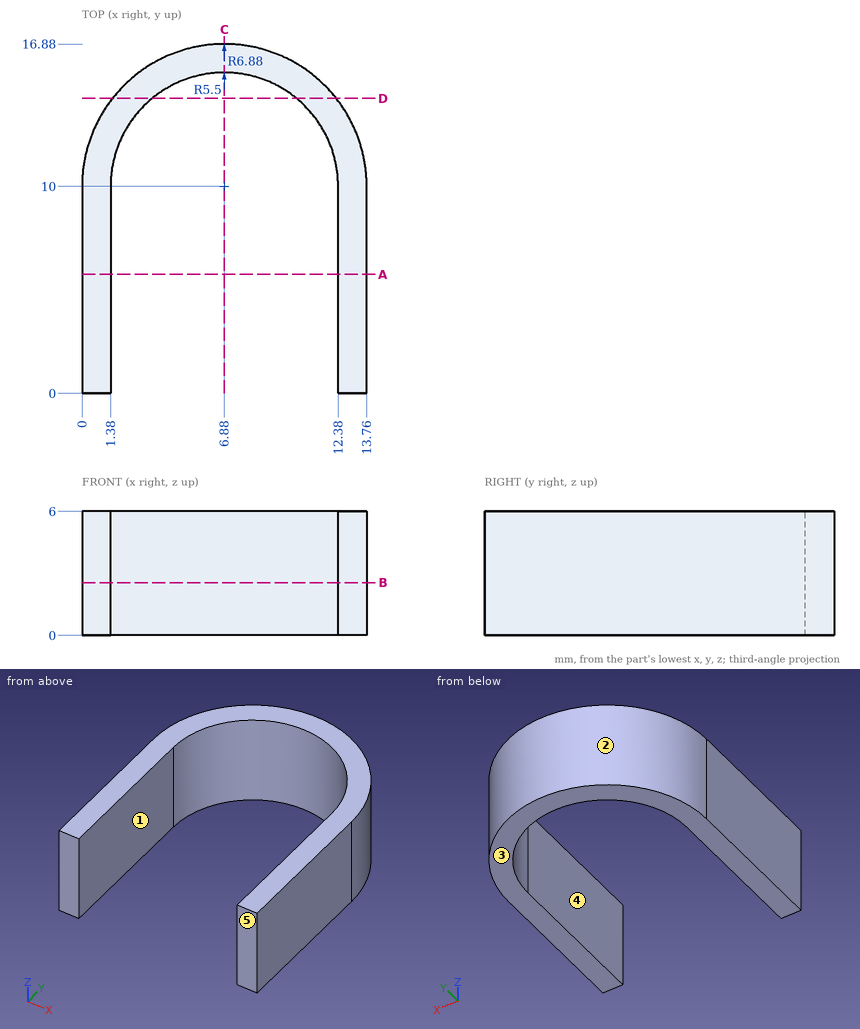
Input: dimensioned drawing with shaded views. Units: mm. Origin: part minimum x, y, z. A direction names the side the tool comes from. Coordinates: 2 decimals unless noted, no trailing zeros. Order: outer loops, then holes, each group sorted by start corner. A loop starts at its lowest first (then second) coordinate and runs counter-clockwise, first axis right, second up. Notation, with made-up numbers: (56, 60.5) -> (108, 60.5) arc R21 cw to (108, 89.5) -> close; hole circle Ø5 at (-6, -26). An arc over 180 degrees is marked (long way). Answer in a Markdown table with one row per item.
Item 1: Section C-C on x = 6.88. Output: boundary loops of the cut face in (y, z).
Return value:
| item | result |
|---|---|
| outline | (15.5, 0) -> (16.88, 0) -> (16.88, 6) -> (15.5, 6) -> close |
Item 2: Contact query for a flat-ended pin moving along its axis: P1, Ø2, axis at x = 10, z = 1, coming from the +Y side. Output: stop coordinate, or through.
Return value:
| item | result |
|---|---|
| P1 | stops at y = 16.55 |
Item 3: Section B-B on z = 2.55. Output: boundary loops of the cut face in (x, y), plus the area to 3 significant figures.
Return value:
| item | result |
|---|---|
| outline | (0, 0) -> (1.38, 0) -> (1.38, 10) arc R5.5 cw to (12.38, 10) -> (12.38, 0) -> (13.76, 0) -> (13.76, 10) arc R6.88 ccw to (0, 10) -> close |
| area | 54.4 mm² |
Item 4: Section D-D on y = 14.25. Output: boundary loops of the cut face in (x, z).
Return value:
| item | result |
|---|---|
| outline | (1.47, 0) -> (3.39, 0) -> (3.39, 6) -> (1.47, 6) -> close; (10.37, 0) -> (12.29, 0) -> (12.29, 6) -> (10.37, 6) -> close |
Item 5: Access query for the marked faces 4 and 5. Directions: +Z, -Z, +X, -X, +Y, -Y. A direction counts if a zero-diameter tool reaches every point of the face in a straight line with its end or side. Return the directions, or none.
Return value:
| item | result |
|---|---|
| face 4 | +Z, -Z, -Y |
| face 5 | +Z, -Z, +X, -X, -Y |
Item 6: Section A-A on y = 5.75. Output: boundary loops of the cut face in (x, z).
Return value:
| item | result |
|---|---|
| outline | (0, 0) -> (1.38, 0) -> (1.38, 6) -> (0, 6) -> close; (12.38, 0) -> (13.76, 0) -> (13.76, 6) -> (12.38, 6) -> close |
Item 7: Draft query along X for the marked faces 1, 2 and 3. Return one class per face: released by +X, released by -X, zero draft, split by the parting line, or undercut.
Return value:
| item | result |
|---|---|
| face 1 | undercut |
| face 2 | split by the parting line |
| face 3 | zero draft |
Item 8: Ray query, L1, parallel to X at y = 4.25, z = 2.25; L2, parallel to X at y = 14.75, z = 4.6; L3, parallel to Y at x = 7, z = 3.75. Return the intervals inside material, ascending.
Return value:
| item | result |
|---|---|
| L1 | x = 0 to 1.38, 12.38 to 13.76 |
| L2 | x = 1.9 to 4.11, 9.65 to 11.86 |
| L3 | y = 15.5 to 16.88 |
